Geometry: final body of the model. Coordinates: model frame, mm. Round coordinates to 2 decimals unless told otherwise and drop trailing zeros. Write each loop counter-clockwise with the first axis right and the second up, starting at its lowest first coordinate (ties: lowest second). Pieces come first, ordered by that corner, then holes. Notation, with made-up numbers: (-36.5, -31) -> (11.5, -31) arc R29 ccw to (11.5, -4) -> close; hole circle Ø5 at (-13, 5.25). An arc over 180 degrees is marked (long way). One line per item, written item: value. Start each with the question number.
from build123d import *

# Parameters (mm, degrees)
F0_R     = 51.5
F1_DEPTH = 7.5
F2_R     = 7.49999
F3_R     = 51.5
F3_R_2   = 44.00001
F4_DEPTH = 7.5
F5_R     = 7.4999
F6_R     = 6
F7_DEPTH = 25


# Not quite as in the source:
# - a fillet or chamfer is up to 0.001 mm smaller than in the source, because OpenCascade refuses the exact size


with BuildPart() as f1:
    # F0 (on Top) → F1 (new body)
    with BuildSketch(Plane.XY):
        Circle(F0_R)
    extrude(amount=F1_DEPTH)

    # F2 (radius 7.5 in the source; OpenCascade refuses exactly that, so slightly less here)
    f2_edges = [f1.edges().sort_by_distance(p)[0] for p in [
        (-51.5, 0, 7.5),
    ]]
    fillet(f2_edges, radius=F2_R)

    # F3 (on face) → F4 (join)
    with BuildSketch(Plane.XY.offset(7.5)):
        Circle(F3_R)
        Circle(F3_R_2, mode=Mode.SUBTRACT)
        Circle(F3_R_2)
    extrude(amount=F4_DEPTH)

    # F5 (radius 7.5 in the source; OpenCascade refuses exactly that, so slightly less here)
    f5_edges = [f1.edges().sort_by_distance(p)[0] for p in [
        (-51.5, 0, 7.5),
    ]]
    fillet(f5_edges, radius=F5_R)

    # F6 (on face) → F7 (cut)
    with BuildSketch(Plane.XY.offset(15)):
        Circle(F6_R)
    extrude(amount=-F7_DEPTH, mode=Mode.SUBTRACT)


solid = f1.part
(1) Line query: probe 1 along Y at (x, z) = (0, 9.25); probe 2 along Y at (x, z) = (0, 12); probe 3 along X at (y, z) = (5, 14.25). Output: solid intervals per line, ascending.
(2) Pin query (flat end, axial travel): pin 1 (2 mm diameter, centred on y = 29.5, z = 3, fed in from +X); pin 2 (4 mm diameter, centred on y = -31, z = 6.5, fed in from -X); pin 3 (15.5 mm diameter, centred on x = 0, y = 0, fed in from +Z); pin 4 (4 mm diameter, centred on x = 2.5, z = 11, fed in from -Y). Return the tip coordinate at first contact, or that it passes through.
(3) Pull-direction query (X, two-part tool) for faces 1 (the face through (-6, 0, 8)), 2 (the face through (-1, -11, 0)); classes: pulls with the +X half, pulls with the -X half, needs draft (parallel to the pull), parting line crosses it, or undercut.
(4) Section query C-C (z = 5.25). Output: boundary loops of the cut face in (x, y), and give its area (3 significant figures).
Results list:
1. probe 1: y = -48.82 to -6, 6 to 48.82
1. probe 2: y = -50.87 to -6, 6 to 50.87
1. probe 3: x = -51.22 to -3.32, 3.32 to 51.22
2. pin 1: stops at x = 42.29
2. pin 2: stops at x = -39.75
2. pin 3: stops at z = 15
2. pin 4: stops at y = -51.17
3. face 1: undercut
3. face 2: needs draft
4. outline: circle Ø98.71 at (0, 0); hole circle Ø12 at (0, 0)
4. area: 7,540 mm^2
